from build123d import *

# Parameters (mm, degrees)
SKETCH2_W                    = 160
SKETCH2_H                    = 70
BASE_FLANGE1_DEPTH           = 3
EDGE_FLANGE1_STRIP_W         = 13.4732
EDGE_FLANGE1_STRIP_H         = 3
EDGE_FLANGE1_STRIP_CUT_DEPTH = 160
EDGE_FLANGE1_DEPTH           = 160


# Sheet-metal steps are written as plain solids
with BuildPart() as part:
    # Sketch2 → Base-Flange1 (new body)
    with BuildSketch(Plane.XY):
        with Locations((-78.670050761, 8.169204738)):
            Rectangle(SKETCH2_W, SKETCH2_H)
        with BuildLine():
            Line((-144.670050761, 33.169204738), (-124.670050761, 33.169204738))
            ThreePointArc((-124.670050761, 33.169204738), (-120.670050761, 29.169204738), (-124.670050761, 25.169204738))
            Line((-124.670050761, 25.169204738), (-144.670050761, 25.169204738))
            ThreePointArc((-144.670050761, 25.169204738), (-148.670050761, 29.169204738), (-144.670050761, 33.169204738))
        make_face(mode=Mode.SUBTRACT)
        with BuildLine():
            Line((-12.670050761, 25.169204738), (-36.670050761, 25.169204738))
            ThreePointArc((-36.670050761, 25.169204738), (-40.670050761, 29.169204738), (-36.670050761, 33.169204738))
            Line((-36.670050761, 33.169204738), (-12.670050761, 33.169204738))
            ThreePointArc((-12.670050761, 33.169204738), (-8.670050761, 29.169204738), (-12.670050761, 25.169204738))
        make_face(mode=Mode.SUBTRACT)
    extrude(amount=-BASE_FLANGE1_DEPTH)

    # Edge-Flange1 strip (across the edge) → Edge-Flange1 strip cut (cut)
    with BuildSketch(Plane(origin=(-158.670050761, -26.830795262, 0), x_dir=(0, 1, 0), z_dir=(1, 0, 0))):
        with Locations((-3, -1.5)):
            Rectangle(EDGE_FLANGE1_STRIP_W, EDGE_FLANGE1_STRIP_H)
    extrude(amount=EDGE_FLANGE1_STRIP_CUT_DEPTH, mode=Mode.SUBTRACT)

    # Edge-Flange1 section (across the edge) → Edge-Flange1 (add)
    with BuildSketch(Plane(origin=(-158.670050761, -26.830795262, 0), x_dir=(0, 1, 0), z_dir=(1, 0, 0))):
        with BuildLine():
            Line((0, 0.7366), (0, 17))
            Line((0, 17), (3, 17))
            Line((3, 17), (3, 0.7366))
            ThreePointArc((3, 0.7366), (3.215745145, 0.215745145), (3.7366, 0))
            Line((3.7366, 0), (3.7366, -3))
            ThreePointArc((3.7366, -3), (1.094424801, -1.905575199), (0, 0.7366))
        make_face()
    extrude(amount=EDGE_FLANGE1_DEPTH)


solid = part.part
Source: CAD feature listing. Evaluate the final solid. Frame: model axes, mm. A direction names the side the tool comes from. Round coordinates to 2 decimals unless told otherwise and drop trailing zeros. Loops run counter-clockwise (first coordinate to the right, second up) from the corner with the lowest first, then second, coordinate; pieces in that order, holes last.
Q1. Section D-D, the plane z = 8.5. Return loops of the section in (x, y).
Q2. Section C-C, the plane y = 11. Return loops of the section in (x, z), plus the area to 3 significant figures.
Q3. Section A-A, the plane x = -15. Return loops of the section in (y, z).
Q4. Ray query, line 1 (Z direction, x = -23, y = 34); line 2 (Y direction, x = -126.5, z = 12.75). Return the intervals inside material, ascending.
Q5. First-contact query: P1, Ø2.5, axis at x = -26, z = -1.5, coming from the -Y side; P2, Ø3, axis at x = -24.5, y = 11, coming from the +Z side; P3, Ø3.5, axis at x = -139, z = -1.5, coming from the -Y side. Flat tips, straight axial feed; report the tip coordinate or a pass-through.
Q6. Section B-B, the plane x = -45. Return loops of the section in (y, z).
Q7. Access query for faces 5 (the face through (-80, -23.831, 9)), 6 (the face through (-80, -25, 17)), 7 (the face through (-25, 33.169, -1)). Directions: +Z, -Z, +X, -X, +Y, -Y. A direction counts if a zero-diameter tool reaches every point of the face in a straight line with its end or side. Return the directions, or none.
Q8. Mould query, pull axis X, two halves, no side actions, for faces 1 (the face through (-80, 11, -3)), 2 (the face through (-135, 25.169, -1)), 3 (the face through (-40.67, 29.08, -1.48)), 4 (the face through (-158.67, 3.1, -0.4)). Classes: pulls with the +X half, pulls with the -X half, needs draft (parallel to the pull), parting line crosses it, or undercut.
Solutions:
1. outline: (-158.67, -26.83) - (1.33, -26.83) - (1.33, -23.83) - (-158.67, -23.83) - close
2. outline: (-158.67, -3) - (1.33, -3) - (1.33, 0) - (-158.67, 0) - close
2. area: 480 mm2
3. outline: (-26.83, 0.74) arc R3.74 ccw to (-23.09, -3) - (25.17, -3) - (25.17, 0) - (-23.09, 0) arc R0.74 cw to (-23.83, 0.74) - (-23.83, 17) - (-26.83, 17) - close; (33.17, -3) - (43.17, -3) - (43.17, 0) - (33.17, 0) - close
4. line 1: z = -3 to 0
4. line 2: y = -26.83 to -23.83
5. P1: stops at y = -26.7
5. P2: stops at z = 0
5. P3: stops at y = -26.8
6. outline: (-26.83, 0.74) arc R3.74 ccw to (-23.09, -3) - (43.17, -3) - (43.17, 0) - (-23.09, 0) arc R0.74 cw to (-23.83, 0.74) - (-23.83, 17) - (-26.83, 17) - close
7. face 5: +Z, +X, -X, +Y
7. face 6: +Z, +X, -X, +Y, -Y
7. face 7: +Z, -Z
8. face 1: needs draft
8. face 2: undercut
8. face 3: undercut
8. face 4: pulls with the -X half
